The model under review builds one solid part; all positions refer to its coordinate system, in mm. A direction names the side the tool comes from. Coordinates: 2 decimals unless noted, no trailing zeros. Order: outer loops, then holes, each group sorted by start corner. A loop starts at its lowest first (then second) coordinate and runs counter-clockwise, first axis right, second up. Notation, with made-up numbers: M 67,-36.5 L 106,-36.5 A16 cw 106,-23.5 Z; hole C 88,-4 d5. An arc over 180 degrees is marked long. One line per item, written item: value.
```python
from build123d import *

# Parameters (mm, degrees)
SKETCH_1_R               = 17.5
EXTRUDE_1_DEPTH          = 25
SKETCH_2_R               = 10
EXTRUDE_2_DEPTH          = 1
SKETCH_3_R               = 13
EXTRUDE_3_DEPTH          = 5
SKETCH_4_R               = 4
CUT_EXTRUDE_1_DEPTH      = 47
SKETCH_5_R               = 1.5
CUT_EXTRUDE_2_DEPTH      = 47
PATTERN_CIRCULAR_1_COUNT = 3
SKETCH_8_R               = 10
CUT_EXTRUDE_3_DEPTH      = 0.1
SKETCH_9_R               = 0.645
EXTRUDE_4_DEPTH          = 20
SKETCH_10_R              = 0.645
EXTRUDE_5_DEPTH          = 10
EXTRUDE_6_DEPTH          = 1.5


with BuildPart() as part:
    # 草图1 → 凸台-拉伸1 (new body)
    with BuildSketch(Plane(origin=(0, 0, 0), x_dir=(1, 0, 0), z_dir=(0, 1, 0))):
        Circle(SKETCH_1_R)
    extrude(amount=EXTRUDE_1_DEPTH)

    # 草图2 → 凸台-拉伸2 (add)
    with BuildSketch(Plane(origin=(0, 25, 0), x_dir=(1, 0, 0), z_dir=(0, 1, 0))):
        Circle(SKETCH_2_R)
    extrude(amount=EXTRUDE_2_DEPTH)

    # 草图3 → 凸台-拉伸3 (add)
    with BuildSketch(Plane(origin=(0, 26, 0), x_dir=(1, 0, 0), z_dir=(0, 1, 0))):
        Circle(SKETCH_3_R)
    extrude(amount=EXTRUDE_3_DEPTH)

    # 草图4 → 切除-拉伸1 (cut)
    with BuildSketch(Plane(origin=(0, 31, 0), x_dir=(1, 0, 0), z_dir=(0, 1, 0))):
        Circle(SKETCH_4_R)
    extrude(amount=-CUT_EXTRUDE_1_DEPTH, mode=Mode.SUBTRACT)

    # 草图5 → 切除-拉伸2 (cut)
    with BuildSketch(Plane(origin=(0, 0, 0), x_dir=(0, 0, -1), z_dir=(1, 0, 0))):
        with Locations((0, 28.5)):
            Circle(SKETCH_5_R)
    cut_extrude_2 = extrude(amount=-CUT_EXTRUDE_2_DEPTH, mode=Mode.SUBTRACT)

    # 阵列(圆周)1: 切除-拉伸2 ×3 about axis
    pattern_circular_1_axis = Axis((0, 39.080777009, 0), (0, -1, 0))
    for i in range(1, PATTERN_CIRCULAR_1_COUNT):
        add(cut_extrude_2.rotate(pattern_circular_1_axis, i * 360 / PATTERN_CIRCULAR_1_COUNT), mode=Mode.SUBTRACT)

    # 草图8 → 切除-拉伸3 (cut)
    with BuildSketch(Plane(origin=(0, 31, 0), x_dir=(1, 0, 0), z_dir=(0, 1, 0))):
        Circle(SKETCH_8_R)
    extrude(amount=-CUT_EXTRUDE_3_DEPTH, mode=Mode.SUBTRACT)

    # 草图9 → 凸台-拉伸4 (add)
    with BuildSketch(Plane(origin=(0, 30.9, 0), x_dir=(1, 0, 0), z_dir=(0, 1, 0))):
        with Locations((-5.423552013, 6.793867644)):
            Circle(SKETCH_9_R)
        with Locations((-4.297718988, 7.443867644)):
            Circle(SKETCH_9_R)
        with Locations((-3.171885963, 8.093867644)):
            Circle(SKETCH_9_R)
        with Locations((-4.773552013, 5.668034619)):
            Circle(SKETCH_9_R)
        with Locations((-3.647718988, 6.318034619)):
            Circle(SKETCH_9_R)
        with Locations((-2.521885963, 6.968034619)):
            Circle(SKETCH_9_R)
    extrude(amount=EXTRUDE_4_DEPTH)

    # 草图10 → 凸台-拉伸5 (add)
    with BuildSketch(Plane.XZ):
        with Locations((0.65, 13.624722325)):
            Circle(SKETCH_10_R)
        with Locations((-0.65, 13.624722325)):
            Circle(SKETCH_10_R)
        with Locations((0, 14.75055535)):
            Circle(SKETCH_10_R)
        with Locations((0.65, -14.375277675)):
            Circle(SKETCH_10_R)
        with Locations((-0.65, -14.375277675)):
            Circle(SKETCH_10_R)
        with Locations((0, -13.24944465)):
            Circle(SKETCH_10_R)
    extrude(amount=EXTRUDE_5_DEPTH)

    # 草图11 → 凸台-拉伸6 (add)
    with BuildSketch(Plane.XZ):
        with BuildLine():
            Line((-26.5, 3), (-21.5, 3))
            ThreePointArc((-21.5, 3), (-18.5, 0), (-21.5, -3))
            Line((-21.5, -3), (-26.5, -3))
            Line((-26.5, -3), (-26.5, -6))
            Line((-26.5, -6), (-11.5, -6))
            Line((-11.5, -6), (-11.5, 6))
            Line((-11.5, 6), (-26.5, 6))
            Line((-26.5, 6), (-26.5, 3))
        make_face()
        with BuildLine():
            Line((11.5, -6), (11.5, 6))
            Line((11.5, 6), (26.5, 6))
            Line((26.5, 6), (26.5, 3))
            Line((26.5, 3), (21.5, 3))
            ThreePointArc((21.5, 3), (18.5, 0), (21.5, -3))
            Line((21.5, -3), (26.5, -3))
            Line((26.5, -3), (26.5, -6))
            Line((26.5, -6), (11.5, -6))
        make_face()
    extrude(amount=EXTRUDE_6_DEPTH)


solid = part.part
```
(1) For L1, parallel to Z at x = 0, y = 13; L2, parallel to Y at x = 7, z = 9, list the stretches that pass through material, from the lowest coordinate up.
Geometry results:
L1: z = -17.5 to -4, 4 to 17.5
L2: y = 0 to 25, 26 to 31
(2) We need section B-B, the plane y = 28.5. State the section outline as (x, z) points, plus the area to 3 significant figures.
Geometry results:
outline: M -12.91,-1.5 A13 ccw 5.16,-11.93 L 0.56,-3.96 A4 cw -3.71,-1.5 Z; M -12.91,1.5 L -3.71,1.5 A4 cw 0.56,3.96 L 5.16,11.93 A13 ccw Z; M 3.15,-2.46 L 7.76,-10.43 A13 ccw 7.76,10.43 L 3.15,2.46 A4 cw Z
area: 399 mm2
(3) We need section C-C, the plane y = 36. State the section outline as (x, z) points (3 decimals).
Geometry results:
outline: C -5.424,-6.794 d1.29; C -4.774,-5.668 d1.29; C -4.298,-7.444 d1.29; C -3.648,-6.318 d1.29; C -3.172,-8.094 d1.29; C -2.522,-6.968 d1.29
(4) We need section A-A, the plane z = 0. Count the separate pieces of the cut face and the enclosed holes in it, plus the area to 3 significant figures.
Geometry results:
separate pieces: 3
enclosed holes: 0
area: 770 mm2
(5) Insertion check: pin 1 Ø0.8 at (x, y) = (-19.5, -0.5) entering from +Z; pin 2 Ø2 at (x, y) = (-8.5, 19.5) entering from +Z; pin 3 Ø13 at (x, z) = (1.5, 3) entering from -Y; pin 4 Ø5 at (x, z) = (0, 0) entering from -Y. Each pin has a flat end and moves straight along its axis. Give the tip position at first contact, or say it passes through.
Geometry results:
pin 1: stops at z = 6
pin 2: stops at z = 15.81
pin 3: stops at y = 0
pin 4: passes through
(6) Mouldability with a two-part tool opening along X and no side actions: class faces 5 (the cylindrical face through (18.5, -0.7, 0.1)), 6 (the flat face through (-0.1, 30.9, 4.3)), 7 (the flat face through (19, -1, -6)), 8 (the flat face through (-11.5, -1, 0)) as +X half, -X half, draft (parallel to the pull), parting line (faces both ways), or undercut.
Geometry results:
face 5: +X half
face 6: undercut
face 7: draft
face 8: undercut
(7) Tool access review of faces 1 (the flat face through (24, -1, -3)), 2 (the flat face through (-19, -1, 6)), 3 (the flat face through (-24, -1, 3)), 4 (the cylindrical face through (-2.17, 25.49, 9.76)): name each direction out of +Z, -Z, +X, -X, +Y, -Y from which nothing blocks a thin tool from reaching the whole face with its end or side.
Geometry results:
face 1: +X, +Y, -Y
face 2: +Z, +X, -X, -Y
face 3: -X, +Y, -Y
face 4: none
